from build123d import *

# Parameters (mm, degrees)
F3_DEPTH     = 4.7762
F4_R         = 4.8895
F5_DEPTH     = 1.6002
F6_R         = 1.905
F7_DEPTH     = 3.1760001
F9_R         = 3.683
F10_DEPTH    = 1.9060001
F11_T1_DEPTH = 2.2381504403


# Not quite as in the source:
# - a fillet or chamfer that OpenCascade refuses, or shapes differently, is made with other operations: its cross-section is extruded or revolved along the edge and cut away or added


with BuildPart() as f1:
    # F0 (on Front) → F1 (revolve)
    with BuildSketch(Plane.XZ):
        with BuildLine():
            Line((9.525, 4.7752), (9.525, 0))
            Line((9.525, 0), (25.4, 0))
            Line((25.4, 0), (25.4, 1.10784454))
            ThreePointArc((25.4, 1.10784454), (24.8095678029, 2.6410913648), (23.343266994, 3.382318687))
            Line((23.343266994, 3.382318687), (9.525, 4.7752))
        make_face()
    revolve(axis=Axis((0, 0, 2.1961550228), (0, 0, 1)))

    # F2 (on face) → F3 (cut, through all)
    with BuildSketch(Plane(origin=(0, 0, 0), x_dir=(1, 0, 0), z_dir=(0, 0, -1))):
        with BuildLine():
            Line((-25.4, 25.4), (-25.4, 0))
            Line((-25.4, 0), (-22.225, 0))
            ThreePointArc((-22.225, 0), (-17.4625, 4.7625), (-12.7, 0))
            Line((-12.7, 0), (-9.525, 0))
            ThreePointArc((-9.525, 0), (0, 9.525), (9.525, 0))
            Line((9.525, 0), (12.7, 0))
            ThreePointArc((12.7, 0), (17.4625, 4.7625), (22.225, 0))
            Line((22.225, 0), (25.4, 0))
            Line((25.4, 0), (25.4, 25.4))
            Line((25.4, 25.4), (-25.4, 25.4))
        make_face()
        with BuildLine():
            ThreePointArc((9.525, 0), (0, 9.525), (-9.525, 0))
            ThreePointArc((-9.525, 0), (0, -9.525), (9.525, 0))
        make_face()
    extrude(amount=-F3_DEPTH, mode=Mode.SUBTRACT)

    # F4 (on face) → F5 (cut)
    with BuildSketch(Plane(origin=(0, 0, 0), x_dir=(1, 0, 0), z_dir=(0, 0, -1))):
        with Locations((-17.4625, 0)):
            Circle(F4_R)
        with Locations((17.4625, 0)):
            Circle(F4_R)
    extrude(amount=-F5_DEPTH, mode=Mode.SUBTRACT)

    # F6 (on face) → F7 (cut, through all)
    with BuildSketch(Plane(origin=(0, 0, 1.6002), x_dir=(1, 0, 0), z_dir=(0, 0, -1))):
        with Locations((-17.4625, 0)):
            Circle(F6_R)
        with Locations((17.4625, 0)):
            Circle(F6_R)
    extrude(amount=-F7_DEPTH, mode=Mode.SUBTRACT)

    # F9 (on offset) → F10 (cut, through all)
    with BuildSketch(Plane(origin=(0, 0, 2.8702), x_dir=(1, 0, 0), z_dir=(0, 0, -1))):
        with Locations((17.4625, 0)):
            Circle(F9_R)
        with Locations((-17.4625, 0)):
            Circle(F9_R)
    extrude(amount=-F10_DEPTH, mode=Mode.SUBTRACT)

    # F11: chamfer of 0.254 on 4 edges, made by hand

    # F11_s2 → F11_t1 (cut)
    with BuildSketch(Plane.XY.offset(-0.6379504403)):
        with BuildLine():
            Line((-22.3460344648, 0.2414567901), (-22.5997245668, 0))
            Line((-22.5997245668, 0), (-22.352, 0))
            ThreePointArc((-22.352, 0), (-22.3504182536, 0.1243599467), (-22.3460344648, 0.2414567901))
        make_face()
        with BuildLine():
            Line((-12.5789655352, 0.2414567901), (-12.3252754332, 0))
            Line((-12.3252754332, 0), (-12.573, 0))
            ThreePointArc((-12.573, 0), (-12.5745817464, 0.1243599467), (-12.5789655352, 0.2414567901))
        make_face()
        with BuildLine():
            Line((12.5789655352, 0.2414567901), (12.3252754332, 0))
            Line((12.3252754332, 0), (12.573, 0))
            ThreePointArc((12.573, 0), (12.5745817464, 0.1243599467), (12.5789655352, 0.2414567901))
        make_face()
        with BuildLine():
            Line((22.3460344648, 0.2414567901), (22.5997245668, 0))
            Line((22.5997245668, 0), (22.352, 0))
            ThreePointArc((22.352, 0), (22.3504182536, 0.1243599467), (22.3460344648, 0.2414567901))
        make_face()
    extrude(amount=F11_T1_DEPTH, mode=Mode.SUBTRACT)


solid = f1.part
The listing builds one solid part. Answer for the finished solid, in the listing's coordinates (mm). A direction names the side the tool comes from. Round coordinates to 2 decimals unless told otherwise and drop trailing zeros. Order: outer loops, then holes, each group sorted by start corner. A loop starts at its lowest first (then second) coordinate and runs counter-clockwise, first axis right, second up. Notation, with made-up numbers: (6, -16.5) - (18, -16.5) arc R29 cw to (18, 6.5) - close; hole circle Ø3 at (-4, 35.25). An arc over 180 degrees is marked (long way). Write item = value, one per line. Start each with the question number.
1) Section A-A, the plane x = 0 is taken. Write down the section's boundary in (y, z) (3 decimals).
2) Given pin 1 (3.5 mm diameter, centred on x = 18.5, y = -1.5, fed in from +Z); pin 2 (5 mm diameter, centred on x = -16.5, y = -2.5, fed in from -Z); pin 3 (2.5 mm diameter, centred on x = 23.5, z = 1, fed in from -Y), each flat-ended and moving along its own axis, determine where each tip first touches the part or whether it passes through.
3) For faces 1 (the flat face through (-24, 0, 2)), 2 (the cylindrical face through (-13.95, -1.11, 3.43)), 3 (the flat face through (11, 0, 2)), determine the directions among +Z, -Z, +X, -X, +Y, -Y from which every point of the face is accessible in a straight line to the end or side of a thin tool.
4) Straight lines are drawn through the part: L1, parallel to Y at x = -11.5, z = 1.5; L2, parallel to Z at x = 10, y = 4; L3, parallel to X at y = 11.5, z = 1.45. For each, find the intervals that lie inside material, in ascending order.
Results list:
q1.outline = (9.525, 0) - (25.4, 0) - (25.4, 1.108) arc R2.286 ccw to (23.343, 3.382) - (9.525, 4.775) - close
q2.pin_1 = 2.87
q2.pin_2 = 1.6
q2.pin_3 = 0
q3.face_1 = +Z, -Z, -X, -Y
q3.face_2 = +Z
q3.face_3 = +Z, -Z, -Y
q4.L1 = 0 to 22.61
q4.L2 = 0 to 4.65
q4.L3 = -22.62 to 22.62
